Check sheet for the modelled part. Datum: model origin and axes. Units: mm. A direction names the side the tool comes from. Round coordinates to 2 decimals unless told otherwise and drop trailing zeros. Order: outer loops, then holes, each group sorted by start corner. A loop starts at its lowest first (then second) coordinate and runs counter-clockwise, first axis right, second up.
from build123d import *

# Parameters (mm, degrees)
F0_W     = 35.56
F0_H     = 35.56
F0_W_2   = 6.35
F0_H_2   = 6.35
F1_DEPTH = 2.286
F2_DEPTH = 20.32
F3_W     = 6.35
F3_H     = 6.35
F4_DEPTH = 12.7
F5_R     = 5.08
F6_R     = 2.54
F7_W     = 6.35
F7_H     = 5.08
F8_DEPTH = 5.08
F9_R     = 1.27


with BuildPart() as f1:
    # F0 (on Front) → F1 (new body)
    with BuildSketch(Plane.XZ):
        Rectangle(F0_W, F0_H)
        Rectangle(F0_W_2, F0_H_2, mode=Mode.SUBTRACT)
    extrude(amount=F1_DEPTH)

    # F0 (on Front) → F2 (join)
    with BuildSketch(Plane.XZ):
        Rectangle(F0_W_2, F0_H_2)
    extrude(amount=F2_DEPTH)

    # F3 (on face) → F4 (join)
    with BuildSketch(Plane.XY.offset(3.175)):
        with Locations((0, -17.145)):
            Rectangle(F3_W, F3_H)
    extrude(amount=F4_DEPTH)

    # F5
    f5_edges = [f1.edges().sort_by_distance(p)[0] for p in [
        (0, -20.32, -3.175),
    ]]
    fillet(f5_edges, radius=F5_R)

    # F6
    f6_edges = [f1.edges().sort_by_distance(p)[0] for p in [
        (3.175, -20.32, 8.89),
        (-3.175, -20.32, 8.89),
    ]]
    fillet(f6_edges, radius=F6_R)

    # F7 (on face) → F8 (join)
    with BuildSketch(Plane(origin=(0, -13.97, 0), x_dir=(-1, 0, 0), z_dir=(0, 1, 0))):
        with Locations((0, 13.335)):
            Rectangle(F7_W, F7_H)
    extrude(amount=F8_DEPTH)

    # F9
    f9_edges = [f1.edges().sort_by_distance(p)[0] for p in [
        (2.431051, -19.576051, 15.875),
        (0, -20.32, 15.875),
        (-2.431051, -19.576051, 15.875),
    ]]
    fillet(f9_edges, radius=F9_R)


solid = f1.part
1) Sectioned sample at B-B on x = -11.5. Record the cut outline in (y, z).
2) Set-up check for faces 5 (the face through (-3.175, -15, 5)), 6 (the face through (2.813, -13.273, 15.493)), 7 (the face through (0, -14, 15.875)), 8 (the face through (3.175, -15, 5)), 9 (the face through (2.41, -8.85, -2.45)): record each of +Z, -Z, +X, -X, +Y, -Y from which the full face is reachable in a straight line by a thin tool's end or side.
3) Sectioned sample at A-A on z = 7. Record the cut outline in (x, y) (3 decimals), and give its area (3 significant figures).
4) Draft check along Y on faces 1 (the face through (0, -8.89, 13)), 2 (the face through (0, -1, 17.78)), 3 (the face through (0.01, -19.96, 15.49)), 4 (the face through (0, -11, 10.795)). Enter one of: pulls with the +Y half, pulls with the -Y half, needs draft (parallel to the pull), parting line crosses it, or undercut.
5) Sectioned sample at C-C on y = -6.25. Record the cut outline in (x, z) (3 decimals).
6) Sectioned sample at D-D on z = -10.5. Record the cut outline in (x, y), and give its area (3 significant figures).
7) Gauge pin test, flat ends, axial feed: pin 1 (1 mm diameter, centred on x = 0, y = -11, fed in from -Z) (3 decimals); pin 2 (3 mm diameter, centred on x = 1, y = -13.5, fed in from +Z) (3 decimals); pin 3 (1 mm diameter, centred on y = -15, z = -1, fed in from +X) (3 decimals). Record the tip position at first contact, or that the pin passes through.
8) Scan lines: line 1 (X direction, y = -4.5, z = 3) (3 decimals); line 2 (Y direction, x = -6, z = -4); line 3 (Y direction, x = -2, z = 11.5). Record each from-to range of solid material in increasing order.
Values found:
1. outline: (-2.29, -17.78) - (0, -17.78) - (0, 17.78) - (-2.29, 17.78) - close
2. face 5: +Z, -Z, -X, -Y
2. face 6: +Z, +X, -Y
2. face 7: +Z, +X, -X, -Y
2. face 8: +Z, -Z, +X, -Y
2. face 9: -Z, +X, -Y
3. outline: (-17.78, -2.286) - (17.78, -2.286) - (17.78, 0) - (-17.78, 0) - close; (-3.175, -17.78) arc R2.54 ccw to (-0.635, -20.32) - (0.635, -20.32) arc R2.54 ccw to (3.175, -17.78) - (3.175, -13.97) - (-3.175, -13.97) - close
3. area: 119 mm2
4. face 1: undercut
4. face 2: needs draft
4. face 3: pulls with the -Y half
4. face 4: undercut
5. outline: (-3.175, -0.635) arc R2.54 ccw to (-0.635, -3.175) - (0.635, -3.175) arc R2.54 ccw to (3.175, -0.635) - (3.175, 3.175) - (-3.175, 3.175) - close
6. outline: (-17.78, -2.29) - (17.78, -2.29) - (17.78, 0) - (-17.78, 0) - close
6. area: 81.3 mm2
7. pin 1: stops at z = -3.175
7. pin 2: stops at z = 15.875
7. pin 3: stops at x = 3.175
8. line 1: x = -3.175 to 3.175
8. line 2: y = -2.29 to 0
8. line 3: y = -19.92 to -8.89, -2.29 to 0
